Work out the finished part from the listing and answer in its coordinate system (mm). A direction names the side the tool comes from. Give positions to 0.01 mm unless a question says otherwise; leave off trailing zeros. Loops run counter-clockwise (first coordinate to the right, second up) from the corner with the lowest first, then second, coordinate; pieces in that order, holes last. Notation, with made-up numbers: M -22,15.5 L 30,15.5 A17 ccw 30,35.5 Z; hole C 77.25,7.25 d6. An arc over 180 degrees is marked long. Answer as a JSON object with one key per item and string values. Group by question number.
```python
from build123d import *

# Parameters (mm, degrees)
ESBO_O1_R                   = 30
RESSALTO_EXTRUS_O1_DEPTH    = 40
FURO_ROSCADO_DE_M81_D       = 6.8
FURO_ROSCADO_DE_M81_DEPTH   = 30
FURO_ROSCADO_DE_M81_TIP     = 2.042926105
FUROS_GUIA_COM_8_0MM1_D     = 8
FUROS_GUIA_COM_8_0MM1_DEPTH = 30
FUROS_GUIA_COM_8_0MM1_TIP   = 2.403442476


with BuildPart() as part:
    # Esboço1 → Ressalto-extrusão1 (new body)
    with BuildSketch(Plane.XY):
        with Locations((0, 235)):
            Circle(ESBO_O1_R)
    extrude(amount=RESSALTO_EXTRUS_O1_DEPTH)

    # Furo roscado de M81
    with Locations(Plane.XY.offset(40)):
        with Locations((-17.320508076, 225), (0, 255), (17.320508076, 225)):
            Hole(FURO_ROSCADO_DE_M81_D / 2, depth=FURO_ROSCADO_DE_M81_DEPTH)
            with Locations((0, 0, -(FURO_ROSCADO_DE_M81_DEPTH + FURO_ROSCADO_DE_M81_TIP / 2))):  # 118° drill point
                Cone(0, FURO_ROSCADO_DE_M81_D / 2, FURO_ROSCADO_DE_M81_TIP, mode=Mode.SUBTRACT)

    # Furos-guia com Ø8.0mm1
    with Locations(Plane.XY.offset(40)):
        with Locations((17.320508076, 245), (-17.320508076, 245)):
            Hole(FUROS_GUIA_COM_8_0MM1_D / 2, depth=FUROS_GUIA_COM_8_0MM1_DEPTH)
            with Locations((0, 0, -(FUROS_GUIA_COM_8_0MM1_DEPTH + FUROS_GUIA_COM_8_0MM1_TIP / 2))):  # 118° drill point
                Cone(0, FUROS_GUIA_COM_8_0MM1_D / 2, FUROS_GUIA_COM_8_0MM1_TIP, mode=Mode.SUBTRACT)


solid = part.part
```
Item 1: A tool of negligible diameter and unlimited length cuts with its end or side. For faces 4 (the flat face through (0, 235, 0)), 5 (the cylindrical face through (-1.828, 257.867, 24.79)), from which of +Z, -Z, +X, -X, +Y, -Y can it reach the whole face along a straight path? Write none if from no direction.
Item 2: A cutting plane is placed at B-B (y = 259.5). Determine the outline of the cut face in (x, z).
Item 3: A cutting plane is placed at A-A (z = 31). Determine the outline of the cut face in (x, y).
Item 4: Given pin 1 Ø10 at (x, z) = (-20.5, 20.5) entering from -Y; pin 2 Ø12 at (x, z) = (6.5, 34.5) entering from -Y; pin 3 Ø4 at (y, z) = (252.5, 21.5) entering from -X, each flat-ended and moving along its own axis, determine where each tip first touches the part or whether it passes through.
Item 5: Find the intervals of material crossed by probe 1 along Y at (x, z) = (-19.5, 31.5); probe 2 along X at (y, z) = (245, 33.5); probe 3 along Y at (x, z) = (0, 29.25), in increasing order. Write a range as [from, to].
Item 6: For a pull along Y with two mould halves and no side action, classify faces 1 (the cylindrical face through (-3.905, 264.745, 19.72)), 2 (the cylindrical face through (15.17, 248.373, 24.79)), 3 (the flat face through (0, 235, 40)) as pulls with the +Y half, pulls with the -Y half, needs draft (parallel to the pull), parting line crosses it, or undercut.
Item 7: A cutting plane is placed at C-C (x = -25). Determine the outline of the cut face in (y, z), and give its area (3 significant figures).
The answers:
{
 "1": {"face 4": "-Z, +X, -X, +Y, -Y", "face 5": "+Z"},
 "2": {"outline": "M -17.31,0 L 17.31,0 L 17.31,40 L -17.31,40 Z"},
 "3": {"outline": "C 0,235 d60; hole C -17.32,245 d8; hole C -17.32,225 d6.8; hole C 0,255 d6.8; hole C 17.32,245 d8; hole C 17.32,225 d6.8"},
 "4": {"pin 1": "stops at y = 209.31", "pin 2": "stops at y = 205", "pin 3": "stops at x = -25.69"},
 "5": {"probe 1": "y = [212.2, 222.39], [227.61, 241.65], [248.35, 257.8]", "probe 2": "x = [-28.28, -21.32], [-13.32, 13.32], [21.32, 28.28]", "probe 3": "y = [205, 251.6], [258.4, 265]"},
 "6": {"face 1": "parting line crosses it", "face 2": "undercut", "face 3": "needs draft"},
 "7": {"outline": "M 218.42,0 L 251.58,0 L 251.58,40 L 218.42,40 Z", "area": "1,330 mm^2"}
}
